Input: part model. Units: mm. Frame: model coordinates. Face numbers are marked on the shaded views. Give positions to 0.01 mm unless a question says otherwise; leave off trailing zeros. Order: outer loops, then holes, each group sorted by start corner. A loop starts at its lowest first (then second) coordinate and runs counter-clockwise, first axis right, second up. Notation, with made-up numbers: (77.5, 28.25) - (90.5, 28.25) arc R23 ccw to (90.5, 39.25) - close; hole circle Ø8 at (64, -6). An arc over 180 degrees is marked (long way). Use a Markdown table: item, result.
from build123d import *

# Parameters (mm, degrees)
F0_R     = 100
F1_DEPTH = 25
F3_D     = 30
F3_DEPTH = 10
F3_TIP   = 9.0129092854


with BuildPart() as f1:
    # F0 (on Top) → F1 (new body)
    with BuildSketch(Plane.XY):
        Circle(F0_R)
    extrude(amount=F1_DEPTH)

    # F3
    with Locations(Plane.XY.offset(25)):
        with Locations((-47.1477657557, 46.5463921428), (-60.8591064811, 0), (-47.1477657557, -47.0274910331), (0, -61.4604838192), (48.1099672616, -47.0274910331), (61.5807585418, 0), (48.1099672616, 46.5463921428), (0, 61.4604838192)):
            Hole(F3_D / 2, depth=F3_DEPTH)
            with Locations((0, 0, -(F3_DEPTH + F3_TIP / 2))):  # 118° drill point
                Cone(0, F3_D / 2, F3_TIP, mode=Mode.SUBTRACT)


solid = f1.part
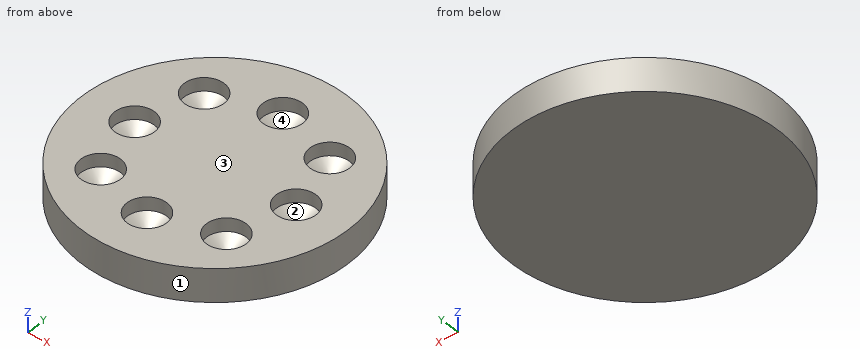
1. Material intervals for line 1 along Y through (x, z) = (0, 21.75); line 2 along Y through (x, z) = (-12, 16.5); line 3 along X through (y, z) = (3.5, 21), sorted ascending.
Response:
| item | result |
|---|---|
| line 1 | y = -100 to -76.46, -46.46 to 46.46, 76.46 to 100 |
| line 2 | y = -99.28 to -70.46, -52.46 to 52.46, 70.46 to 99.28 |
| line 3 | x = -99.94 to -75.45, -46.27 to 46.99, 76.17 to 99.94 |
2. Section query B-B (y = 86). Return loops of the section in (x, z), then the cut area to 3 significant figures.
Response:
| item | result |
|---|---|
| outline | (-51.03, 0) - (51.03, 0) - (51.03, 25) - (-51.03, 25) - close |
| area | 2,550 mm^2 |
3. Section query A-A (z = 11). State how many separate pieces and enclosed holes the cut face has, then the cut area to 3 significant figures.
Response:
| item | result |
|---|---|
| separate pieces | 1 |
| enclosed holes | 8 |
| area | 29,700 mm^2 |
4. Mould query, pull axis Y, two halves, no side actions, for the marked faces 1, 2, 3 and 4. Classes: pulls with the +Y half, pulls with the -Y half, needs draft (parallel to the pull), parting line crosses it, or undercut.
Response:
| item | result |
|---|---|
| face 1 | parting line crosses it |
| face 2 | undercut |
| face 3 | needs draft |
| face 4 | undercut |
5. Pin query (flat end, axial travel): pin 1 (6 mm diameter, centred on y = 12, z = 17, fed in from +X); pin 2 (24 mm diameter, centred on x = -47.15, y = 46.55, fed in from +Z); pin 3 (5 mm diameter, centred on x = -61.5, z = 14, fed in from +Y). Return the tip coordinate at first contact, or that it passes through.
Response:
| item | result |
|---|---|
| pin 1 | stops at x = 99.59 |
| pin 2 | stops at z = 13.2 |
| pin 3 | stops at y = 80.74 |
